from build123d import *

# Parameters (mm, degrees)
SKETCH1_W           = 88.9
SKETCH1_H           = 88.9
BOSS_EXTRUDE1_DEPTH = 8.89
SKETCH2_W           = 25.4
SKETCH2_H           = 21.59
SKETCH2_W_2         = 21.59
SKETCH2_H_2         = 25.4
CUT_EXTRUDE1_DEPTH  = 4.572
SKETCH3_R           = 2.400000026
CUT_EXTRUDE2_DEPTH  = 9.89
SKETCH4_R           = 1.8034
CUT_EXTRUDE3_DEPTH  = 5.318
SKETCH5_R           = 6.35
CUT_EXTRUDE4_DEPTH  = 9.89


with BuildPart() as part:
    # Sketch1 → Boss-Extrude1 (new body)
    with BuildSketch(Plane(origin=(0, 0, 0), x_dir=(1, 0, 0), z_dir=(0, 1, 0))):
        with Locations((44.45, 44.45)):
            Rectangle(SKETCH1_W, SKETCH1_H)
    extrude(amount=BOSS_EXTRUDE1_DEPTH)

    # Sketch2 → Cut-Extrude1 (cut)
    with BuildSketch(Plane(origin=(0, 8.89, 0), x_dir=(1, 0, 0), z_dir=(0, 1, 0))):
        with Locations((44.45, 78.105)):
            Rectangle(SKETCH2_W, SKETCH2_H)
        with Locations((10.795, 44.45)):
            Rectangle(SKETCH2_W_2, SKETCH2_H_2)
        with Locations((44.45, 10.795)):
            Rectangle(SKETCH2_W, SKETCH2_H)
        with Locations((78.105, 44.45)):
            Rectangle(SKETCH2_W_2, SKETCH2_H_2)
    extrude(amount=-CUT_EXTRUDE1_DEPTH, mode=Mode.SUBTRACT)

    # Sketch3 → Cut-Extrude2 (cut, through all)
    with BuildSketch(Plane(origin=(0, 8.89, 0), x_dir=(1, 0, 0), z_dir=(0, 1, 0))):
        with Locations((28.194, 44.45)):
            Circle(SKETCH3_R)
        with Locations((44.45, 60.706)):
            Circle(SKETCH3_R)
        with Locations((60.706, 44.45)):
            Circle(SKETCH3_R)
        with Locations((44.45, 28.194)):
            Circle(SKETCH3_R)
    extrude(amount=-CUT_EXTRUDE2_DEPTH, mode=Mode.SUBTRACT)

    # Sketch4 → Cut-Extrude3 (cut, through all)
    with BuildSketch(Plane(origin=(0, 4.318, 0), x_dir=(1, 0, 0), z_dir=(0, 1, 0))):
        with Locations((75.0062, 52.3875)):
            Circle(SKETCH4_R)
        with Locations((75.0062, 36.5125)):
            Circle(SKETCH4_R)
        with Locations((52.3875, 75.0062)):
            Circle(SKETCH4_R)
        with Locations((36.5125, 75.0062)):
            Circle(SKETCH4_R)
        with Locations((13.8938, 52.3875)):
            Circle(SKETCH4_R)
        with Locations((13.8938, 36.5125)):
            Circle(SKETCH4_R)
        with Locations((36.5125, 13.8938)):
            Circle(SKETCH4_R)
        with Locations((52.3875, 13.8938)):
            Circle(SKETCH4_R)
    extrude(amount=-CUT_EXTRUDE3_DEPTH, mode=Mode.SUBTRACT)

    # Sketch5 → Cut-Extrude4 (cut, through all)
    with BuildSketch(Plane(origin=(0, 8.89, 0), x_dir=(1, 0, 0), z_dir=(0, 1, 0))):
        with Locations((44.45, 44.45)):
            Circle(SKETCH5_R)
    extrude(amount=-CUT_EXTRUDE4_DEPTH, mode=Mode.SUBTRACT)


solid = part.part
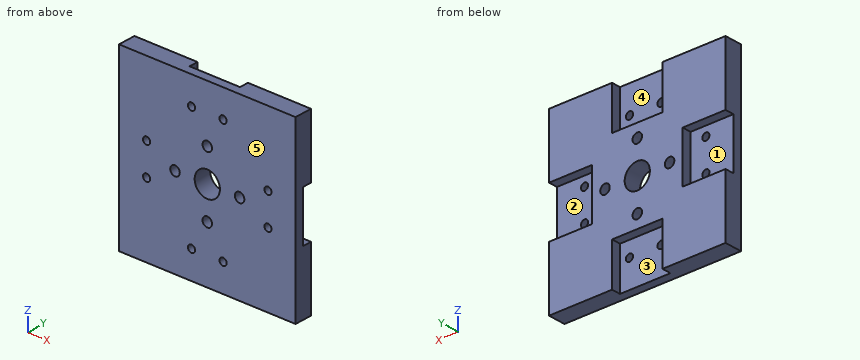
Read the model definition and answer for the solid it produces. Units are mm, in the model's axes. Face numbers are marked on the shaded views. A direction names the side the tool comes from. Round coordinates to 2 decimals unless told otherwise and drop trailing zeros. Loops run counter-clockwise (first coordinate to the right, second up) from the corner with the lowest first, then second, coordinate; pieces in that order, holes last.
Q1. Which of the six approach directions +Z, -Z, +X, -X, +Y, -Y give full straight-line access (tool end or side, diameter ignored) to the marked faces 1, 2 and 3?
Q2. Section D-D on y = 6 is taken. Write down the section's boundary in (x, z), and give its area (3 significant figures).
Q3. Each of these flat-tipped pins is pushed along its axis until it touches: pin 1 (17.5 mm diameter, centred on x = 81.5, z = -44, fed in from +Y); pin 2 (1.4 mm diameter, centred on y = 6.5, z = -41, fed in from +X); pin 3 (1.4 mm diameter, centred on x = 43, y = 7.5, fed in from -Z). Where does it stop, or does it pass through?
Q4. Section C-C on z = -11 is taken. Write down the section's boundary in (x, y).
Q5. Section B-B on x = 44.45 is taken. Write down the section's boundary in (y, z).
Q6. Determine the mould class of the marked faces 4 and 5 for opening direction X: released by +X, released by -X, zero draft, split by the parting line, or undercut.
Q7. Consider probe 1 along Z at (x, y) = (44.45, 6.5); probe 2 along X at (y, z) = (4.5, -44.45); probe 3 along X at (y, z) = (3.25, -44.45). Determine where each line is inside the solid, lowest interval first.
Q8. Section A-A on z = -44.45 is taken. Write down the section's boundary in (x, y), and give its area (3 significant figures).
Output:
1. face 1: -X, +Y
1. face 2: +X, +Y
1. face 3: -Z, +Y
2. outline: (0, -88.9) - (31.75, -88.9) - (31.75, -67.31) - (57.15, -67.31) - (57.15, -88.9) - (88.9, -88.9) - (88.9, -57.15) - (67.31, -57.15) - (67.31, -31.75) - (88.9, -31.75) - (88.9, 0) - (57.15, 0) - (57.15, -21.59) - (31.75, -21.59) - (31.75, 0) - (0, 0) - (0, -31.75) - (21.59, -31.75) - (21.59, -57.15) - (0, -57.15) - close; hole circle Ø4.8 at (28.19, -44.45); hole circle Ø12.7 at (44.45, -44.45); hole circle Ø4.8 at (44.45, -60.71); hole circle Ø4.8 at (44.45, -28.19); hole circle Ø4.8 at (60.71, -44.45)
2. area: 5,510 mm2
3. pin 1: stops at y = 4.32
3. pin 2: stops at x = 67.31
3. pin 3: stops at z = -67.31
4. outline: (0, 0) - (88.9, 0) - (88.9, 8.89) - (57.15, 8.89) - (57.15, 4.32) - (31.75, 4.32) - (31.75, 8.89) - (0, 8.89) - close
5. outline: (0, -88.9) - (4.32, -88.9) - (4.32, -67.31) - (8.89, -67.31) - (8.89, -63.11) - (0, -63.11) - close; (0, -58.31) - (8.89, -58.31) - (8.89, -50.8) - (0, -50.8) - close; (0, -38.1) - (8.89, -38.1) - (8.89, -30.59) - (0, -30.59) - close; (0, -25.79) - (8.89, -25.79) - (8.89, -21.59) - (4.32, -21.59) - (4.32, 0) - (0, 0) - close
6. face 4: undercut
6. face 5: zero draft
7. probe 1: z = -67.31 to -63.11, -58.31 to -50.8, -38.1 to -30.59, -25.79 to -21.59
7. probe 2: x = 21.59 to 25.79, 30.59 to 38.1, 50.8 to 58.31, 63.11 to 67.31
7. probe 3: x = 0 to 25.79, 30.59 to 38.1, 50.8 to 58.31, 63.11 to 88.9
8. outline: (0, 0) - (25.79, 0) - (25.79, 8.89) - (21.59, 8.89) - (21.59, 4.32) - (0, 4.32) - close; (30.59, 0) - (38.1, 0) - (38.1, 8.89) - (30.59, 8.89) - close; (50.8, 0) - (58.31, 0) - (58.31, 8.89) - (50.8, 8.89) - close; (63.11, 0) - (88.9, 0) - (88.9, 4.32) - (67.31, 4.32) - (67.31, 8.89) - (63.11, 8.89) - close
8. area: 395 mm2
